Geometry check sheet. Reference: the model listing, model coordinates, mm. A direction names the side the tool comes from. Give positions to 0.01 mm unless a question says otherwise; leave off trailing zeros. Order: outer loops, then holes, each group sorted by start corner. A loop starts at its lowest first (then second) coordinate and runs counter-clockwise, first axis right, second up. Notation, with made-up numbers: M 36,33 L 59,33 A25 cw 59,69 Z; hole C 66,67.5 d2. An arc over 180 degrees is marked long. Answer as CSV lines item,"result".
from build123d import *

# Parameters (mm, degrees)
SKETCH_2_R      = 22.5
EXTRUDE_1_DEPTH = 30
FILLET_1_R      = 10
SHELL_1_T       = -1
SKETCH_3_R      = 5
EXTRUDE_2_DEPTH = 1


with BuildPart() as part:
    # 草图2 → 凸台-拉伸1 (new body)
    with BuildSketch(Plane(origin=(0, 0, 0), x_dir=(1, 0, 0), z_dir=(0, 1, 0))):
        with Locations(Location((0, 0, 0), (0, 0, 270))):
            Circle(SKETCH_2_R)
    extrude(amount=EXTRUDE_1_DEPTH)

    # 圆角1
    fillet_1_edges = [part.edges().sort_by_distance(p)[0] for p in [
        (0, 30, -22.5),
    ]]
    fillet(fillet_1_edges, radius=FILLET_1_R)

    # 抽壳1
    shell_1_openings = [part.faces().sort_by_distance(p)[0] for p in [
        (0, 0, 0),
    ]]
    offset(amount=SHELL_1_T, openings=shell_1_openings, kind=Kind.INTERSECTION)

    # 草图3 → 凸台-拉伸2 (add)
    with BuildSketch(Plane(origin=(0, 0, 0), x_dir=(1, 0, 0), z_dir=(0, 1, 0))):
        with BuildLine():
            Line((-21.213203436, 7.5), (-30, 7.5))
            ThreePointArc((-30, 7.5), (-37.5, 0), (-30, -7.5))
            Line((-30, -7.5), (-21.213203436, -7.5))
            ThreePointArc((-21.213203436, -7.5), (-22.5, 0), (-21.213203436, 7.5))
        make_face()
        with Locations(Location((-30, 0, 0), (0, 0, 270))):
            Circle(SKETCH_3_R, mode=Mode.SUBTRACT)
    extrude_2 = extrude(amount=EXTRUDE_2_DEPTH)

    # 镜向1: 凸台-拉伸2 across plane
    add(extrude_2.mirror(Plane(origin=(0, 0, 0), x_dir=(0, 0, 1), z_dir=(1, 0, 0))))


solid = part.part
(1) Section check A-A on z = 0. Enter the section's corners in (x, y), then the cut area to 3 significant figures.
The answers:
outline,"M -37.5,0 L -35,0 L -35,1 L -37.5,1 Z; M -25,0 L -21.5,0 L -21.5,20 A9 cw -12.5,29 L 12.5,29 A9 cw 21.5,20 L 21.5,0 L 25,0 L 25,1 L 22.5,1 L 22.5,20 A10 ccw 12.5,30 L -12.5,30 A10 ccw -22.5,20 L -22.5,1 L -25,1 Z; M 35,0 L 37.5,0 L 37.5,1 L 35,1 Z"
area,"105 mm2"
(2) Section check C-C on x = 33.5. Enter the section's corners in (y, z).
The answers:
outline,"M 0,-6.63 L 1,-6.63 L 1,-3.57 L 0,-3.57 Z; M 0,3.57 L 1,3.57 L 1,6.63 L 0,6.63 Z"
(3) Section check B-B on x = 0. Enter the section's corners in (y, z).
The answers:
outline,"M 0,-22.5 L 20,-22.5 A10 ccw 30,-12.5 L 30,12.5 A10 ccw 20,22.5 L 0,22.5 L 0,21.5 L 20,21.5 A9 cw 29,12.5 L 29,-12.5 A9 cw 20,-21.5 L 0,-21.5 Z"
(4) Gauge pin test, flat ends, axial feed: P1, Ø0.8, axis at x = -27.5, y = 0.5, coming from the +Z side; P2, Ø0.8, axis at x = 26, y = 0.5, coming from the -Z side; P3, Ø12, axis at x = 31, z = -3, coming from the +Y side. Record the tip position at first contact, or that the pin passes through.
The answers:
P1,"stops at z = 7.5"
P2,"stops at z = -7.5"
P3,"stops at y = 1"
(5) Section check D-D on y = 13. Enter the section's corners in (x, z).
The answers:
outline,"C 0,0 d45; hole C 0,0 d43"
(6) Tool access check on faces 4 (the face through (14.531, 9.86, -15.846)), 5 (the face through (34.88, 0.49, -1.08)). Record the directions out of +Z, -Z, +X, -X, +Y, -Y that give a thin tool (end or side, any length) a straight path to the whole face; none if there is none.
The answers:
face 4,"-Y"
face 5,"+Y, -Y"
(7) Material ranges on line 1 (X direction, y = 0.4, z = 0); line 2 (Z direction, x = 0, y = 6); line 3 (Z direction, x = 30, y = 0.3), recorded low to high.
The answers:
line 1,"x = -37.5 to -35, -25 to -21.5, 21.5 to 25, 35 to 37.5"
line 2,"z = -22.5 to -21.5, 21.5 to 22.5"
line 3,"z = -7.5 to -5, 5 to 7.5"
(8) Draft check along Z on faces 1 (the face through (0, 30, 0)), 2 (the face through (0, 29, 0)), 3 (the face through (-8.618, 9.86, 20.784)). Enter one of: +Z half, -Z half, draft (parallel to the pull), parting line (faces both ways), or undercut.
The answers:
face 1,"draft"
face 2,"undercut"
face 3,"parting line"
